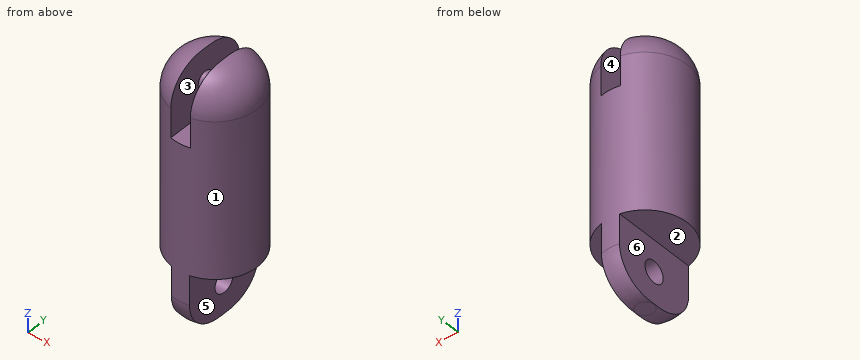
```python
from build123d import *

# Parameters (mm, degrees)
SKETCH1_R           = 100
BOSS_EXTRUDE1_DEPTH = 600
FILLET2_R           = 80
SKETCH2_W           = 46
SKETCH2_H           = 231.861905776
CUT_EXTRUDE1_DEPTH  = 150
SKETCH3_R           = 20.155129503
BOSS_EXTRUDE2_DEPTH = 30
CUT_EXTRUDE2_DEPTH  = 150
FILLET3_R           = 80
SKETCH5_R           = 25.736273229
CUT_EXTRUDE3_DEPTH  = 520


with BuildPart() as part:
    # Sketch1 → Boss-Extrude1 (new body)
    with BuildSketch(Plane.XY):
        Circle(SKETCH1_R)
    extrude(amount=BOSS_EXTRUDE1_DEPTH)

    # Fillet2
    fillet2_edges = [part.edges().sort_by_distance(p)[0] for p in [
        (-100, 0, 600),
    ]]
    fillet(fillet2_edges, radius=FILLET2_R)

    # Sketch2 → Cut-Extrude1 (cut)
    with BuildSketch(Plane.XY.offset(600)):
        Rectangle(SKETCH2_W, SKETCH2_H)
    extrude(amount=-CUT_EXTRUDE1_DEPTH, mode=Mode.SUBTRACT)

    # Sketch3 → Boss-Extrude2 (add, symmetric)
    with BuildSketch(Plane(origin=(0, 0, 0), x_dir=(0, 0, -1), z_dir=(1, 0, 0))):
        with Locations(Location((-524.951093161, 0, 0), (0, 0, 180))):
            Circle(SKETCH3_R)
    extrude(amount=BOSS_EXTRUDE2_DEPTH, both=True)

    # Sketch4 → Cut-Extrude2 (cut)
    with BuildSketch(Plane(origin=(0, 0, 0), x_dir=(-1, 0, 0), z_dir=(0, 0, -1))):
        with BuildLine():
            ThreePointArc((-21.514315111, 97.658252315), (-100, 0), (-21.514315111, -97.658252315))
            Line((-21.514315111, -97.658252315), (-21.514315111, 97.658252315))
        make_face()
        with BuildLine():
            Line((21.514315111, 97.658252315), (21.514315111, -97.658252315))
            ThreePointArc((21.514315111, -97.658252315), (100, 0), (21.514315111, 97.658252315))
        make_face()
    extrude(amount=-CUT_EXTRUDE2_DEPTH, mode=Mode.SUBTRACT)

    # Fillet3
    # the kernel refuses this fillet: 80 mm, written as the material it takes off along each edge
    with BuildSketch(Plane(origin=(0, 0, 0), x_dir=(-0.7984359735160296, 0.6020797257801578, 0), z_dir=(0.6020797257801578, 0.7984359735160296, 0))) as fillet3_piece_1:
        with BuildLine():
            CenterArc((100 - FILLET3_R, FILLET3_R), FILLET3_R, 270, 90)
            Line((100 - FILLET3_R, 0), (100, 0))
            Line((100, 0), (100, FILLET3_R))
        make_face()
    revolve(axis=Axis((0, 0, 0), (0, 0, 1)), revolution_arc=254.037985384, mode=Mode.SUBTRACT)
    with BuildSketch(Plane(origin=(0, 0, 0), x_dir=(0.79843597351603, -0.6020797257801573, 0), z_dir=(-0.6020797257801573, -0.79843597351603, 0))) as fillet3_piece_2:
        with BuildLine():
            CenterArc((100 - FILLET3_R, FILLET3_R), FILLET3_R, 270, 90)
            Line((100 - FILLET3_R, 0), (100, 0))
            Line((100, 0), (100, FILLET3_R))
        make_face()
    revolve(axis=Axis((0, 0, 0), (0, 0, 1)), revolution_arc=254.037985384, mode=Mode.SUBTRACT)

    # Sketch5 → Cut-Extrude3 (cut)
    with BuildSketch(Plane(origin=(21.514315111, 0, 0), x_dir=(0, 0, -1), z_dir=(1, 0, 0))):
        with Locations((-75, 0)):
            Circle(SKETCH5_R)
    extrude(amount=-CUT_EXTRUDE3_DEPTH, mode=Mode.SUBTRACT)


solid = part.part
```
For this review, take the finished solid that the model builds, in its own axes (mm). Face numbers are marked on the shaded views. A direction names the side the tool comes from. Coordinates: 2 decimals unless noted, no trailing zeros. Write each loop counter-clockwise with the first axis right and the second up, starting at its lowest first coordinate (ties: lowest second). Pieces come first, ordered by that corner, then holes.
(1) For pin 1 Ø1 at (x, y) = (-3.5, -12.5) entering from +Z; pin 2 Ø4 at (y, z) = (50, 354.5) entering from +X; pin 3 Ø23.5 at (x, y) = (65, 16) entering from -Z, all flat-tipped, find the tip position at first contact; note any pin that passes through.
(2) Tool access review of the marked faces 5 and 6: name each direction out of +Z, -Z, +X, -X, +Y, -Y from which nothing blocks a thin tool from reaching the whole face with its end or side.
(3) The part is to be moulded in two halves that separate along X. For the marked faces 1, 2, 3 and 4, say which applies: +X half, -X half, draft (parallel to the pull), parting line (faces both ways), or undercut.
(4) Add section A-A on x = 0. Count the separate pieces of the cut face and the enclosed holes in it, then the cut area to 3 significant figures.
(5) Wall thickness on probe 1 along X at (y, z) = (3, 465.5); probe 2 along X at (y, z) = (-13, 545.5); probe 3 along Y at (x, z) = (-3, 244.5): over which ranges is each line inside the solid? List them lowest first.
(6) Add section C-C on z = 397.5. Give the boundary of the cut face in (x, y), then the cut area to 3 significant figures.
Answer sheet:
1. pin 1: stops at z = 541.14
1. pin 2: stops at x = 87.73
1. pin 3: stops at z = 150
2. face 5: -Z, +X, +Y, -Y
2. face 6: -Z, -X, +Y, -Y
3. face 1: parting line
3. face 2: draft
3. face 3: undercut
3. face 4: undercut
4. separate pieces: 2
4. enclosed holes: 1
4. area: 86,400 mm2
5. probe 1: x = -99.95 to -23, 23 to 99.95
5. probe 2: x = -94.94 to -23, 23 to 94.94
5. probe 3: y = -99.95 to 99.95
6. outline: circle Ø200 at (0, 0)
6. area: 31,400 mm2
